Geometry: final body of the model. Coordinates: model frame, mm. A direction names the side the tool comes from. Round coordinates to 2 decimals unless told otherwise and drop trailing zeros. Write each loop counter-clockwise with the first axis right and the second up, starting at its lowest first coordinate (ties: lowest second). Pieces come first, ordered by that corner, then holes. Notation, with made-up numbers: (-9, 67.5) -> (45, 67.5) arc R20 cw to (45, 99.5) -> close; hole circle Ø3 at (82.25, 7). An arc over 180 degrees is marked (long way). Use one line per item in the form item = value. Start each with the question number.
1. Reachability of faces 4 (the face through (-61, 19, -35.75)), 5 (the face through (-60, 37, 0)) from +Z, -Z, +X, -X, +Y, -Y: full face, straight path, thin tool, end or side. Return the list, or none.
2. Draft query along Z for faces 1 (the face through (17, 27, 34.95)), 2 (the face through (25, 19, 1)), 3 (the face through (-61, 19, 35.75)). Return one class per face: pulls with the +Z half, pulls with the -Z half, needs draft (parallel to the pull), parting line crosses it, or undercut.
3. Cut plane B-B, the plane z = -9.5. Return the cut outline in (x, y).
4. Pin query (flat end, axial travel): pin 1 Ø1.5 at (y, z) = (4.5, 14.5) entering from -X. Return the tip coordinate at first contact, or that it passes through.
5. Line query: L1, parallel to X at y = 1, z = 0; L2, parallel to Y at x = 11.5, z = 12; L3, parallel to Z at x = -73.5, y = 26.5. Output: solid intervals per line, ascending.
6. Cut plane C-C, the plane y = 16. Return the cut outline in (x, z).
7. Cut plane A-A, the plane x = -113. Return the cut outline in (y, z).
```python
from build123d import *

# Parameters (mm, degrees)
SKETCH1_W            = 50
SKETCH1_H            = 71.5
BOSS_EXTRUDE1_DEPTH  = 2
SKETCH2_W            = 23
SKETCH2_H            = 12.5
CUT_EXTRUDE1_DEPTH   = 3
SKETCH3_R            = 1.25
CUT_EXTRUDE2_DEPTH   = 3
SKETCH14_W           = 120
SKETCH14_H           = 71.5
BOSS_EXTRUDE7_DEPTH  = 2
SKETCH15_W           = 170
SKETCH15_H           = 1.5
BOSS_EXTRUDE8_DEPTH  = 37.5
SKETCH16_W           = 1.8
SKETCH16_H           = 68.5
BOSS_EXTRUDE9_DEPTH  = 37.5
SKETCH17_W           = 168.2
SKETCH17_H           = 5.5
CUT_EXTRUDE3_DEPTH   = 0.7
SKETCH18_W           = 10.5
SKETCH18_H           = 2.75
CUT_EXTRUDE4_DEPTH   = 1
FILLET4_R            = 2
SKETCH19_W           = 68.5
SKETCH19_H           = 2.5
BOSS_EXTRUDE10_DEPTH = 168.2
CHAMFER1_SIZE        = 0.5


with BuildPart() as part:
    # Sketch1 → Boss-Extrude1 (new body)
    with BuildSketch(Plane(origin=(0, 0, 0), x_dir=(1, 0, 0), z_dir=(0, 1, 0))):
        Rectangle(SKETCH1_W, SKETCH1_H)
    extrude(amount=BOSS_EXTRUDE1_DEPTH)

    # Sketch2 → Cut-Extrude1 (cut)
    with BuildSketch(Plane(origin=(0, 2, 0), x_dir=(1, 0, 0), z_dir=(0, 1, 0))):
        Rectangle(SKETCH2_W, SKETCH2_H)
    extrude(amount=-CUT_EXTRUDE1_DEPTH, mode=Mode.SUBTRACT)

    # Sketch3 → Cut-Extrude2 (cut)
    with BuildSketch(Plane(origin=(0, 2, 0), x_dir=(1, 0, 0), z_dir=(0, 1, 0))):
        with Locations(Location((-13.9, 0, 0), (0, 0, 270))):
            Circle(SKETCH3_R)
        with Locations(Location((13.9, 0, 0), (0, 0, 270))):
            Circle(SKETCH3_R)
    extrude(amount=-CUT_EXTRUDE2_DEPTH, mode=Mode.SUBTRACT)

    # Sketch14 → Boss-Extrude7 (add)
    with BuildSketch(Plane.XZ):
        with Locations((-85, 0)):
            Rectangle(SKETCH14_W, SKETCH14_H)
    extrude(amount=-BOSS_EXTRUDE7_DEPTH)

    # Sketch15 → Boss-Extrude8 (add)
    with BuildSketch(Plane(origin=(0, 2, 0), x_dir=(1, 0, 0), z_dir=(0, 1, 0))):
        with Locations((-60, -35)):
            Rectangle(SKETCH15_W, SKETCH15_H)
        with Locations((-60, 35)):
            Rectangle(SKETCH15_W, SKETCH15_H)
    extrude(amount=BOSS_EXTRUDE8_DEPTH)

    # Sketch16 → Boss-Extrude9 (add)
    with BuildSketch(Plane(origin=(0, 2, 0), x_dir=(1, 0, 0), z_dir=(0, 1, 0))):
        with Locations((24.1, 0)):
            Rectangle(SKETCH16_W, SKETCH16_H)
    extrude(amount=BOSS_EXTRUDE9_DEPTH)

    # Sketch17 → Cut-Extrude3 (cut)
    with BuildSketch(Plane(origin=(0, 0, 34.25), x_dir=(-1, 0, 0), z_dir=(0, 0, -1))):
        with Locations((60.9, 27.25)):
            Rectangle(SKETCH17_W, SKETCH17_H)
    extrude(amount=-CUT_EXTRUDE3_DEPTH, mode=Mode.SUBTRACT)

    # Sketch18 → Cut-Extrude4 (cut)
    with BuildSketch(Plane(origin=(0, 0, 34.95), x_dir=(-1, 0, 0), z_dir=(0, 0, -1))):
        with Locations((-4.95, 28.625)):
            Rectangle(SKETCH18_W, SKETCH18_H)
        with Locations((-4.95, 25.875)):
            Rectangle(SKETCH18_W, SKETCH18_H)
    extrude(amount=-CUT_EXTRUDE4_DEPTH, mode=Mode.SUBTRACT)

    # Fillet4
    fillet4_edges = [part.edges().sort_by_distance(p)[0] for p in [
        (10.2, 24.5, 35.35),
        (10.2, 30, 35.35),
        (-0.3, 30, 35.35),
        (-0.3, 24.5, 35.35),
    ]]
    fillet(fillet4_edges, radius=FILLET4_R)

    # Sketch19 → Boss-Extrude10 (add)
    with BuildSketch(Plane.ZY.offset(-23.2)):
        with Locations((0, 38.25)):
            Rectangle(SKETCH19_W, SKETCH19_H)
    extrude(amount=BOSS_EXTRUDE10_DEPTH)

    # Chamfer1
    chamfer1_edges = [part.edges().sort_by_distance(p)[0] for p in [
        (-60.9, 30, 34.25),
    ]]
    chamfer(chamfer1_edges, length=CHAMFER1_SIZE)


solid = part.part
```
Outcome:
q1.face_4 = -Z, +X, -X, +Y, -Y
q1.face_5 = -X
q2.face_1 = undercut
q2.face_2 = needs draft
q2.face_3 = pulls with the +Z half
q3.outline = (-145, 0) -> (25, 0) -> (25, 39.5) -> (-145, 39.5) -> (-145, 37) -> (23.2, 37) -> (23.2, 2) -> (-145, 2) -> close
q4.pin_1 = 23.2
q5.L1 = -145 to -15.15, -12.65 to -11.5, 11.5 to 12.65, 15.15 to 25
q5.L2 = 0 to 2, 37 to 39.5
q5.L3 = -35.75 to -34.25, 34.95 to 35.75
q6.outline = (-145, -35.75) -> (25, -35.75) -> (25, 35.75) -> (-145, 35.75) -> (-145, 34.25) -> (23.2, 34.25) -> (23.2, -34.25) -> (-145, -34.25) -> close
q7.outline = (0, -35.75) -> (39.5, -35.75) -> (39.5, 35.75) -> (0, 35.75) -> close; hole (2, -34.25) -> (37, -34.25) -> (37, 34.25) -> (30.5, 34.25) -> (30, 34.75) -> (30, 34.95) -> (24.5, 34.95) -> (24.5, 34.25) -> (2, 34.25) -> close
